Part model, mm, in its own coordinate system. A direction names the side the tool comes from. Give positions to 0.01 mm unless a question says otherwise; leave off trailing zeros. Order: outer loops, then holes, each group sorted by start corner. A loop starts at its lowest first (then second) coordinate and runs counter-clockwise, first axis right, second up. Notation, with made-up numbers: (50, 89) -> (105, 89) arc R24 cw to (105, 105) -> close; hole circle Ø6 at (47.5, 1.5). An arc over 180 degrees is marked (long way). Write item = value, one per line. Start each with the question number.
Item 1: Tool access for faces 1 (the face through (-66.514, 31.225, 13.172)), 2 (the face through (46, 13.75, 16)): list every direction of +Z, -Z, +X, -X, +Y, -Y with a clear straight run to the whole face (end or side of a thin tool).
Item 2: Band-saw the part on A-A on z = 2.5. Write the cut outline in (x, y).
Item 3: Drill centre lines: line 1 along Y through (x, z) = (-66.15, 10); line 2 along X through (y, z) = (4.5, 10.5); line 3 along X through (y, z) = (-23, 14.5). Where is each one in solid material? Low to high.
Item 4: Band-saw the part on D-D on x = 63. Write the cut outline in (y, z).
Item 5: Flat gauge pins, fed straight in: P1, Ø3, axis at x = -33.5, y = 22.5, coming from the -Z side; P2, Ø3.5, axis at x = 38.5, y = 31, coming from the -Z side. Where does each tip first touch, or does it go through?
Item 6: Band-saw the part on C-C on x = -3. Write the cut outline in (y, z), plus the area to 3 significant figures.
Item 7: Pull direction Y, two halves, no side cores. Call faces 3 (the face through (-21, 31, 18)), 4 (the face through (0, 35, 0)): +Y half, -Y half, draft (parallel to the pull), parting line (faces both ways), or undercut.
```python
from build123d import *

# Parameters (mm, degrees)
SKETCH3_W            = 135
SKETCH3_H            = 72.5
BOSS_EXTRUDE1_DEPTH  = 20
SKETCH4_W            = 131
SKETCH4_H            = 68.5
CUT_EXTRUDE1_DEPTH   = 18
SKETCH6_W            = 23
SKETCH6_H            = 45.9
BOSS_EXTRUDE2_DEPTH  = 8
SKETCH5_W            = 21.8
SKETCH5_H            = 43.5
CUT_EXTRUDE2_DEPTH   = 18
SKETCH7_W            = 1.2
SKETCH7_H            = 8.3
SKETCH7_H_2          = 11.3
BOSS_EXTRUDE5_DEPTH  = 8
SKETCH9_W            = 1.2
SKETCH9_H            = 65.5
BOSS_EXTRUDE6_DEPTH  = 8
SKETCH11_W           = 26.8
SKETCH11_H           = 36
BOSS_EXTRUDE7_DEPTH  = 8
SKETCH10_W           = 25.6
SKETCH10_H           = 33.6
CUT_EXTRUDE3_DEPTH   = 8
SKETCH13_W           = 8
SKETCH13_H           = 33.6
CUT_EXTRUDE4_DEPTH   = 1.2
SKETCH14_R           = 3.9
CUT_EXTRUDE5_DEPTH   = 2
SKETCH15_R           = 5.9
CUT_EXTRUDE6_DEPTH   = 2
SKETCH18_W           = 5
SKETCH18_H           = 5
BOSS_EXTRUDE8_DEPTH  = 5
SKETCH19_R           = 1.5
CUT_EXTRUDE7_DEPTH   = 8
SKETCH20_W           = 5
SKETCH20_H           = 5
BOSS_EXTRUDE9_DEPTH  = 5
SKETCH21_R           = 1.5
CUT_EXTRUDE8_DEPTH   = 5
SKETCH23_W           = 7
SKETCH23_H           = 7
BOSS_EXTRUDE10_DEPTH = 5
SKETCH24_R           = 1.5
CUT_EXTRUDE10_DEPTH  = 5


with BuildPart() as part:
    # Sketch3 → Boss-Extrude1 (new body)
    with BuildSketch(Plane.XY):
        Rectangle(SKETCH3_W, SKETCH3_H)
    extrude(amount=BOSS_EXTRUDE1_DEPTH)

    # Sketch4 → Cut-Extrude1 (cut)
    with BuildSketch(Plane(origin=(0, 0, 0), x_dir=(-1, 0, 0), z_dir=(0, 0, -1))):
        Rectangle(SKETCH4_W, SKETCH4_H)
    extrude(amount=-CUT_EXTRUDE1_DEPTH, mode=Mode.SUBTRACT)

    # Sketch6 → Boss-Extrude2 (add)
    with BuildSketch(Plane(origin=(0, 0, 18), x_dir=(-1, 0, 0), z_dir=(0, 0, -1))):
        with Locations((-54, 0)):
            Rectangle(SKETCH6_W, SKETCH6_H)
    extrude(amount=BOSS_EXTRUDE2_DEPTH)

    # Sketch5 → Cut-Extrude2 (cut)
    with BuildSketch(Plane(origin=(0, 0, 18), x_dir=(-1, 0, 0), z_dir=(0, 0, -1))):
        with Locations((-54.6, 0)):
            Rectangle(SKETCH5_W, SKETCH5_H)
    extrude(amount=CUT_EXTRUDE2_DEPTH, mode=Mode.SUBTRACT)

    # Sketch7 → Boss-Extrude5 (add)
    with BuildSketch(Plane(origin=(0, 0, 18), x_dir=(-1, 0, 0), z_dir=(0, 0, -1))):
        with Locations((-43.1, -27.1)):
            Rectangle(SKETCH7_W, SKETCH7_H)
        with Locations((-43.1, 28.6)):
            Rectangle(SKETCH7_W, SKETCH7_H_2)
    extrude(amount=BOSS_EXTRUDE5_DEPTH)

    # Sketch9 → Boss-Extrude6 (add)
    with BuildSketch(Plane(origin=(0, 0, 18), x_dir=(-1, 0, 0), z_dir=(0, 0, -1))):
        with Locations((25.55, 1.5)):
            Rectangle(SKETCH9_W, SKETCH9_H)
    extrude(amount=BOSS_EXTRUDE6_DEPTH)

    # Sketch11 → Boss-Extrude7 (add)
    with BuildSketch(Plane(origin=(0, 0, 18), x_dir=(-1, 0, 0), z_dir=(0, 0, -1))):
        with Locations((39.55, 0)):
            Rectangle(SKETCH11_W, SKETCH11_H)
    extrude(amount=BOSS_EXTRUDE7_DEPTH)

    # Sketch10 → Cut-Extrude3 (cut)
    with BuildSketch(Plane(origin=(0, 0, 18), x_dir=(-1, 0, 0), z_dir=(0, 0, -1))):
        with Locations((38.95, 0)):
            Rectangle(SKETCH10_W, SKETCH10_H)
    extrude(amount=CUT_EXTRUDE3_DEPTH, mode=Mode.SUBTRACT)

    # Sketch13 → Cut-Extrude4 (cut)
    with BuildSketch(Plane.ZY.offset(52.95)):
        with Locations((14, 0)):
            Rectangle(SKETCH13_W, SKETCH13_H)
    extrude(amount=-CUT_EXTRUDE4_DEPTH, mode=Mode.SUBTRACT)

    # Sketch14 → Cut-Extrude5 (cut)
    with BuildSketch(Plane(origin=(67.5, 0, 0), x_dir=(0, 0, -1), z_dir=(1, 0, 0))):
        with Locations((-10, -28.45)):
            Circle(SKETCH14_R)
    extrude(amount=-CUT_EXTRUDE5_DEPTH, mode=Mode.SUBTRACT)

    # Sketch15 → Cut-Extrude6 (cut)
    with BuildSketch(Plane.ZY.offset(67.5)):
        with Locations((10, 26.25)):
            Circle(SKETCH15_R)
        with Locations((10, 6.25)):
            Circle(SKETCH15_R)
        with Locations((10, -13.75)):
            Circle(SKETCH15_R)
    extrude(amount=-CUT_EXTRUDE6_DEPTH, mode=Mode.SUBTRACT)

    # Sketch18 → Boss-Extrude8 (add)
    with BuildSketch(Plane(origin=(0, 0, 18), x_dir=(-1, 0, 0), z_dir=(0, 0, -1))):
        with Locations((39.55, -14.3)):
            Rectangle(SKETCH18_W, SKETCH18_H)
        with Locations((39.55, 14.3)):
            Rectangle(SKETCH18_W, SKETCH18_H)
    extrude(amount=BOSS_EXTRUDE8_DEPTH)

    # Sketch19 → Cut-Extrude7 (cut)
    with BuildSketch(Plane(origin=(0, 0, 10), x_dir=(-1, 0, 0), z_dir=(0, 0, -1))):
        with Locations((39.663798911, -14.3)):
            Circle(SKETCH19_R)
        with Locations((39.663798911, 14.3)):
            Circle(SKETCH19_R)
    extrude(amount=-CUT_EXTRUDE7_DEPTH, mode=Mode.SUBTRACT)

    # Sketch20 → Boss-Extrude9 (add)
    with BuildSketch(Plane(origin=(0, 0, 18), x_dir=(-1, 0, 0), z_dir=(0, 0, -1))):
        with Locations((-46.2, 16.25)):
            Rectangle(SKETCH20_W, SKETCH20_H)
        with Locations((-63, -16.25)):
            Rectangle(SKETCH20_W, SKETCH20_H)
    extrude(amount=BOSS_EXTRUDE9_DEPTH)

    # Sketch21 → Cut-Extrude8 (cut)
    with BuildSketch(Plane(origin=(0, 0, 13), x_dir=(-1, 0, 0), z_dir=(0, 0, -1))):
        with Locations((-46.2, 16.25)):
            Circle(SKETCH21_R)
        with Locations((-63, -16.25)):
            Circle(SKETCH21_R)
    extrude(amount=-CUT_EXTRUDE8_DEPTH, mode=Mode.SUBTRACT)

    # Sketch23 → Boss-Extrude10 (add)
    with BuildSketch(Plane(origin=(0, 0, 18), x_dir=(-1, 0, 0), z_dir=(0, 0, -1))):
        with Locations((-39, 30.75)):
            Rectangle(SKETCH23_W, SKETCH23_H)
        with Locations((21.45, 30.75)):
            Rectangle(SKETCH23_W, SKETCH23_H)
        with Locations((21.45, -27.75)):
            Rectangle(SKETCH23_W, SKETCH23_H)
        with Locations((-39, -27.75)):
            Rectangle(SKETCH23_W, SKETCH23_H)
    extrude(amount=BOSS_EXTRUDE10_DEPTH)

    # Sketch24 → Cut-Extrude10 (cut)
    with BuildSketch(Plane(origin=(0, 0, 13), x_dir=(-1, 0, 0), z_dir=(0, 0, -1))):
        with Locations((-39, 30.75)):
            Circle(SKETCH24_R)
        with Locations((21.45, 30.75)):
            Circle(SKETCH24_R)
        with Locations((21.45, -27.75)):
            Circle(SKETCH24_R)
        with Locations((-39, -27.75)):
            Circle(SKETCH24_R)
    extrude(amount=-CUT_EXTRUDE10_DEPTH, mode=Mode.SUBTRACT)


solid = part.part
```
Values found:
q1.face_1 = -X
q1.face_2 = -Z
q2.outline = (-67.5, -36.25) -> (67.5, -36.25) -> (67.5, 36.25) -> (-67.5, 36.25) -> close; hole (-65.5, -34.25) -> (65.5, -34.25) -> (65.5, 34.25) -> (-65.5, 34.25) -> close
q3.line_1 = -36.25 to -19.65, -7.85 to 0.35, 12.15 to 20.35, 32.15 to 36.25
q3.line_2 = -26.15 to -24.95, 42.5 to 43.7, 65.5 to 67.5
q3.line_3 = -67.5 to -65.5, -26.15 to -24.95, 42.5 to 43.7, 65.5 to 67.5
q4.outline = (-36.25, 0) -> (-34.25, 0) -> (-34.25, 18) -> (-22.95, 18) -> (-22.95, 10) -> (-21.75, 10) -> (-21.75, 18) -> (-18.75, 18) -> (-18.75, 13) -> (-17.75, 13) -> (-17.75, 18) -> (-14.75, 18) -> (-14.75, 13) -> (-13.75, 13) -> (-13.75, 18) -> (21.75, 18) -> (21.75, 10) -> (22.95, 10) -> (22.95, 18) -> (34.25, 18) -> (34.25, 0) -> (36.25, 0) -> (36.25, 20) -> (-36.25, 20) -> close
q5.P1 = 18
q5.P2 = 13
q6.outline = (-36.25, 0) -> (-34.25, 0) -> (-34.25, 18) -> (34.25, 18) -> (34.25, 0) -> (36.25, 0) -> (36.25, 20) -> (-36.25, 20) -> close
q6.area = 217 mm^2
q7.face_3 = undercut
q7.face_4 = draft
